```python
from build123d import *

# Parameters (mm, degrees)
F0_W      = 15
F0_H      = 63.5
F1_DEPTH  = 1
F2_W      = 15
F2_H      = 100
F3_DEPTH  = 1
F5_DEPTH  = 15
F7_D      = 3.7973
F7_DEPTH  = 1.0010001
F8_D      = 3.7973
F8_DEPTH  = 99.0010001
F9_D      = 3.7973
F10_R     = 3
F12_DEPTH = 15


# Not quite as in the source:
# - the dataset's text gives a spline's control points without its knots; the knots are read off the source's solid


with BuildPart() as f1:
    # F0 (on Front) → F1 (new body)
    with BuildSketch(Plane.XZ):
        with Locations((0, -31.75)):
            Rectangle(F0_W, F0_H)
    extrude(amount=F1_DEPTH)

    # F2 (on Top) → F3 (join)
    with BuildSketch(Plane.XY):
        with Locations((0, -50)):
            Rectangle(F2_W, F2_H)
    extrude(amount=-F3_DEPTH)

    # F4 (on face) → F5 (join, through all)
    with BuildSketch(Plane.YZ.offset(7.5)):
        with BuildLine():
            add(Edge.make_bspline(
                [(-1, -59.1678209603), (-4.7628395259, -45.3067980707), (-29.7762758586, -17.4602950514), (-61.8860200047, -5.5842199363), (-92.6793441176, -1)],
                knots=[0, 0, 0, 0, 0.4491979362, 1, 1, 1, 1], degree=3))
            Line((-1, -59.1678209603), (-0.1314357545, -58.9320325989))
            add(Edge.make_bspline(
                [(-0.1314357545, -58.9320325989), (-1.2015793269, -54.989987117), (-3.6884016693, -49.2559925066), (-8.3530917512, -42.083257521), (-12.4261382193, -36.9661666224), (-16.9750747913, -32.1385398724), (-21.9011436861, -27.6279890298), (-27.1107997825, -23.4618046647), (-32.4934625877, -19.6712415186), (-38.1217352473, -16.235966274), (-44.0944999552, -13.1322911599), (-50.5030405646, -10.3365734857), (-59.7536135039, -6.9863101985), (-72.8745679903, -3.4418665365), (-85.5418056788, -1.1526510188), (-92.5468210682, -0.109810334)],
                knots=[0, 0, 0, 0, 0.125, 0.1875, 0.25, 0.3125, 0.375, 0.4375, 0.5, 0.5625, 0.625, 0.6875, 0.75, 0.875, 1, 1, 1, 1], degree=3))
            Line((-92.5468210682, -0.109810334), (-92.6793441176, -1))
        make_face()
    extrude(amount=-F5_DEPTH)

    # F7 (through all, one way)
    with BuildSketch(Plane.XZ.offset(1)):
        with Locations((0, -12.3973852023)):
            Circle(F7_D / 2)
    extrude(amount=-F7_DEPTH, mode=Mode.SUBTRACT)

    # F8 (through all, one way)
    with BuildSketch(Plane(origin=(0, -1, 0), x_dir=(1, 0, 0), z_dir=(0, 1, 0))):
        with Locations((0, 42.5568334758)):
            Circle(F8_D / 2)
    extrude(amount=-F8_DEPTH, mode=Mode.SUBTRACT)

    # F9 (through all)
    with Locations(Plane.XZ.offset(1)):
        with Locations((0, -42.5568334758)):
            Hole(F9_D / 2)

    # F10
    f10_edges = [f1.edges().sort_by_distance(p)[0] for p in [
        (0, -1, -1),
    ]]
    fillet(f10_edges, radius=F10_R)

    # F11 (on face) → F12 (join, through all)
    with BuildSketch(Plane.YZ.offset(7.5)):
        with BuildLine():
            Line((-100, -1), (-100, 0))
            ThreePointArc((-100, 0), (-105.5726686693, -3.7761825834), (-104.1308658813, -10.3515453659))
            Line((-104.1308658813, -10.3515453659), (-103.4423882344, -9.6262878049))
            ThreePointArc((-103.4423882344, -9.6262878049), (-104.6438905577, -4.1468188195), (-100, -1))
        make_face()
    extrude(amount=-F12_DEPTH)


solid = f1.part
```
Part model, mm, in its own coordinate system. A direction names the side the tool comes from. Coordinates: 2 decimals unless noted, no trailing zeros. Write item = value, one per line. Start each with the question number.
Item 1: Cut at A-A, the plane x = 0. State how many separate pieces and enclosed holes the cut face has, and give its area (3 significant figures).
Item 2: 3-axis set-ups, long thin cutter, end or side, ignore diameter. For faces 4 (the flat face through (0, -1, -61)), 5 (the cylindrical face through (-0.247, -0.507, -10.515)), 6 (the cylindrical face through (-0.11, -1.9, -1.86)): which of +Z, -Z, +X, -X, +Y, -Y reach the whole face in a straight line?
Item 3: Wall check: L1, parallel to Z at x = 0, y = -0.25; L2, parallel to Z at x = 0, y = -9.25; L3, parallel to Y at x = -1.75, z = -37. Give the ranges that are in metal, low to high. Write a range as from..to.
Item 4: Mould opens along Z. For faces 1 (the flat face through (0, -49, 0)), 2 (the cylindrical face through (0.105, -104.674, -4.225)), 3 (the flat face through (0, -96, -1)) say: released by +Z, released by -Z, zero draft, split by the parting line, or undercut.
Item 5: Flat gauge pins, fed straight in: pin 1 Ø5 at (y, z) = (-15.5, -31.5) entering from +X; pin 2 Ø5 at (x, z) = (0, -42.56) entering from -Y; pin 3 Ø2.5 at (x, z) = (0, -12.4) entering from +Y; pin 4 Ø3 at (x, z) = (-2, -36.5) entering from -Y. Where does each tip first touch, or does it go through?
The answers:
q1.separate_pieces = 3
q1.enclosed_holes = 0
q1.area = 265 mm2
q2.face_4 = -Z, +X, -X, -Y
q2.face_5 = +Y
q2.face_6 = +X, -X
q3.L1 = -63.5..-44.46, -40.66..-14.3, -10.5..0
q3.L2 = -1..0
q3.L3 = -13.71..-12.52, -1..0
q4.face_1 = released by +Z
q4.face_2 = undercut
q4.face_3 = released by -Z
q5.pin_1 = 7.5
q5.pin_2 = -11.14
q5.pin_3 = -43.2
q5.pin_4 = -15.55
